Autodesk Inventor part; units mm, degrees
ref_plane "YZ Plane" through (0, 0, 0) normal (1, 0, 0) x (0, 1, 0)
ref_plane "XY Plane" through (0, 0, 0) normal (0, 0, 1) x (1, 0, 0)
sketch "Sketch1" plane through (0, 0, 0) normal (0, 0, 1) x (1, 0, 0)
  line L0 (0, 0) -> (609.6, 0)
  line L1 (609.6, 0) -> (609.6, 317.881)
  line L2 (609.6, 317.881) -> (0, 317.881)
  line L3 (0, 317.881) -> (0, 0)
  dimension "d0" = 609.6
  dimension "d1" = 317.881
extrude "Extrusion1" add sketch "Sketch1" along normal blind 5.7658
sketch "Sketch2" plane through (0, 317.881, 0) normal (0, 1, 0) x (1, 0, 0)
  line L0 (609.6, 0) -> (0, 0)
  line L1 (0, 0) -> (0, -5.7658)
  line L2 (609.6, -5.7658) -> (0, -5.7658)
  line L3 (609.6, 0) -> (609.6, -5.7658)
  line L4 (0, 0) -> (609.6, 0)
  line L5 (0, 0) -> (14.4594, -5.7658)
  line L6 (0, -5.7658) -> (609.6, -5.7658)
  line L7 (14.4594, -5.7658) -> (14.4594, 0)
  line L8 (14.4594, -5.7658) -> (20.2252, -5.7658) construction
  dimension "d4" = 21.74
  dimension "d5" = 90
extrude "Extrusion2" cut sketch "Sketch2" against normal through all contours L5 L2 L1
sketch "Sketch3" plane through (609.6, 0, 0) normal (1, 0, 0) x (0, 0, -1)
  line L0 (0, 0) -> (0, 317.881)
  line L1 (0, 317.881) -> (-5.7658, 317.881)
  line L2 (-5.7658, 0) -> (-5.7658, 317.881)
  line L3 (0, 0) -> (-5.7658, 0)
  line L4 (0, 0) -> (-5.7658, 0)
  line L5 (0, 0) -> (-5.7658, 5.7658)
  line L6 (-5.7658, 0) -> (-5.7658, 317.881)
  line L7 (0, 0) -> (8.1541, 0) construction
  line L8 (0, 317.881) -> (-5.7658, 317.881)
  line L9 (0, 317.881) -> (-5.7658, 312.1152)
  line L10 (0, 317.881) -> (8.1541, 317.881) construction
  dimension "d8" = 135
  dimension "d9" = 135
extrude "Extrusion3" cut sketch "Sketch3" against normal through all contours L3 L2 L5 | L9 L2 L1
ref_plane "Center Plane" through (0, 158.9405, 0) normal (0, 1, 0) x (-1, 0, 0)
sketch "Sketch4" plane through (0, 158.9405, 0) normal (0, 1, 0) x (-1, 0, 0)
  line L0 (-14.4594, 5.7658) -> (0, 0)
  line L1 (-609.6, 5.7658) -> (-14.4594, 5.7658)
  line L2 (-609.6, 0) -> (-609.6, 5.7658)
  line L3 (-609.6, 0) -> (0, 0)
  line L4 (-609.6, 5.7658) -> (-584.2, 5.7658) construction
  line L5 (-609.6, 5.7658) -> (-14.4594, 5.7658) construction
  line L6 (-584.2, 5.7658) -> (-609.6, 4.4413)
  point P0 (0, 0)
  dimension "d13" = 25.4
  dimension "d14" = 2.985
extrude "Extrusion4" cut sketch "Sketch4" against normal through all both and the other way through all contours L6 L2 L1
sketch "Sketch5" plane through (0, 0, 5.7658) normal (0, 0, 1) x (1, 0, 0)
  line L0 (97.0094, 261.3152) -> (501.65, 261.3152)
  line L1 (527.05, 235.9152) -> (527.05, 81.9658)
  line L2 (501.65, 56.5658) -> (97.0094, 56.5658)
  line L3 (71.6094, 81.9658) -> (71.6094, 235.9152)
  line L4 (584.2, 312.1152) -> (14.4594, 312.1152)
  line L5 (14.4594, 5.7658) -> (584.2, 5.7658)
  line L6 (584.2, 5.7658) -> (584.2, 312.1152)
  line L7 (14.4594, 312.1152) -> (14.4594, 5.7658)
  arc A0 (97.0094, 261.3152) -> (71.6094, 235.9152) centre (97.0094, 235.9152) ccw
  arc A1 (527.05, 235.9152) -> (501.65, 261.3152) centre (501.65, 235.9152) ccw
  arc A2 (501.65, 56.5658) -> (527.05, 81.9658) centre (501.65, 81.9658) ccw
  arc A3 (71.6094, 81.9658) -> (97.0094, 56.5658) centre (97.0094, 81.9658) ccw
  point P0 (0, 0)
  dimension "d18" = 50.8
  dimension "d19" = 50.8
  dimension "d20" = 57.15
  dimension "d21" = 57.15
  dimension "d22" = 25.4
extrude "Extrusion5" cut sketch "Sketch5" against normal through all contours L0 A1 L1 A2 L2 A3 L3 A0
sketch "Sketch6" plane through (0, 0, 5.7658) normal (0, 0, 1) x (1, 0, 0)
  circle A0 centre (539.75, 56.5658) radius 2.7559
  circle A1 centre (539.75, 132.7658) radius 2.7559
  circle A2 centre (539.75, 185.1152) radius 2.75
  circle A3 centre (539.75, 261.3152) radius 2.7559
  line L0 (527.05, 235.9152) -> (527.05, 81.9658)
  line L1 (501.65, 56.5658) -> (97.0094, 56.5658)
  circle A4 centre (58.9026, 56.5658) radius 2.7559
  circle A5 centre (58.9026, 132.7658) radius 2.7559
  circle A6 centre (58.9026, 185.1152) radius 2.75
  circle A7 centre (58.9026, 261.3152) radius 2.7559
  circle A8 centre (476.25, 47.6758) radius 2.7559
  circle A9 centre (374.65, 47.6758) radius 2.7559
  circle A10 centre (224.0026, 47.6758) radius 2.7559
  circle A11 centre (122.4026, 47.6758) radius 2.7559
  circle A12 centre (476.25, 270.2052) radius 2.7559
  circle A13 centre (374.65, 270.2052) radius 2.7559
  circle A14 centre (224.0026, 270.2052) radius 2.7559
  circle A15 centre (122.4026, 270.2052) radius 2.7559
  point P0 (0, 0)
  dimension "d25" = 5.5118
  dimension "d26" = 5.5118
  dimension "d27" = 5.5
  dimension "d28" = 5.5118
  dimension "d29" = 12.7
  dimension "d30" = 25.4
  dimension "d31" = 76.2
  dimension "d32" = 52.3494
  dimension "d33" = 76.2
  dimension "d34" = 12.7
  dimension "d35" = 12.7
  dimension "d36" = 12.7
  dimension "d39" = 480.8474
  dimension "d44" = 5.5118
  dimension "d45" = 5.5118
  dimension "d46" = 5.5118
  dimension "d48" = 63.5
  dimension "d49" = 8.89
  dimension "d50" = 8.89
  dimension "d51" = 8.89
  dimension "d53" = 101.6
  dimension "d54" = 150.6474
  dimension "d55" = 5.5118
  dimension "d56" = 101.6
  dimension "d57" = 8.89
  dimension "d63" = 222.5294
extrude "Extrusion6" cut sketch "Sketch6" against normal through all
properties part number "Wind Tunnel Test Section Front" material "Polycarbonate, Clear"
Work out the finished part from the listing and answer in its coordinate system (mm). A direction names the side the tool comes from. Give positions to 0.01 mm unless a question says otherwise; leave off trailing zeros. Order: outer loops, then holes, each group sorted by start corner. A loop starts at its lowest first (then second) coordinate and runs counter-clockwise, first axis right, second up.
1. Straight lines are drawn through the part: L1, parallel to Y at x = 374.65, z = 2.75; L2, parallel to Y at x = 175, z = 1.85; L3, parallel to Y at x = 316.5, z = 4.85. For each, find the intervals that lie inside material, in ascending order.
Result sheet:
L1: y = 2.75 to 44.92, 50.43 to 56.57, 261.32 to 267.45, 272.96 to 315.13
L2: y = 1.85 to 56.57, 261.32 to 316.03
L3: y = 4.85 to 56.57, 261.32 to 313.03
2. For faces 1 (the flat face through (596.722, 161.103, 5.113)), 2 (the cylindrical face through (519.4, 63.8, 2.9)), determine the directions among +Z, -Z, +X, -X, +Y, -Y from which every point of the face is accessible in a straight line to the end or side of a thin tool.
Result sheet:
face 1: +Z, +X, +Y, -Y
face 2: +Z, -Z
3. Section B-B, the plane y = 227.5 is taken. Determine the outline of the cut face in (x, z).
Result sheet:
outline: (0, 0) - (71.61, 0) - (71.61, 5.77) - (14.46, 5.77) - close; (527.05, 0) - (609.6, 0) - (609.6, 4.44) - (584.2, 5.77) - (527.05, 5.77) - close
4. Section C-C, the plane z = 1.85 is taken. Give the number of separate pieces and of enclosed holes in the cut face, and give its area (3 significant figures).
Result sheet:
separate pieces: 1
enclosed holes: 17
area: 97,000 mm2
5. This flat-tipped pin is pushed along its axis until it touches: P1, Ø4.5, axis at x = 58.9, y = 56.57, coming from the +Z side. Where does it stop, or does it pass through?
Result sheet:
P1: passes through
6. Section D-D, the plane y = 73 is taken. Determine the outline of the cut face in (x, z), and give its area (3 significant figures).
Result sheet:
outline: (0, 0) - (73.24, 0) - (73.24, 5.77) - (14.46, 5.77) - close; (525.41, 0) - (609.6, 0) - (609.6, 4.44) - (584.2, 5.77) - (525.41, 5.77) - close
area: 849 mm2
7. The mould has two halves that part along Y. Classify faces 3 (the cylindrical face through (519.807, 253.677, 2.923)), 4 (the cylindrical face through (78.852, 64.204, 2.923)), 5 (the flat face through (7.128, 161.166, 2.843)): released by +Y, released by -Y, zero draft, split by the parting line, or undercut.
Result sheet:
face 3: undercut
face 4: undercut
face 5: zero draft
8. Section A-A, the plane x = 460 is taken. Determine the outline of the cut face in (y, z).
Result sheet:
outline: (0, 0) - (56.57, 0) - (56.57, 5.77) - (5.77, 5.77) - close; (261.32, 0) - (317.88, 0) - (312.12, 5.77) - (261.32, 5.77) - close
